```python
from build123d import *

# Parameters (mm, degrees)
F0_W     = 103.351444006
F0_H     = 32.4089471251
F0_R     = 8.8186134511
F2_DEPTH = 23.876
F3_T     = 2.54
F4_R     = 5.08
F5_DEPTH = 75.946
F6_DEPTH = 25.4


# Not quite as in the source:
# - a shell that OpenCascade refuses in one call is made with other operations: the cavity is built on its own and cut out
# - the program builds the solid bodies; features that only make, move or delete a surface that nothing else refers to are left out


with BuildPart() as f2:
    # F0 (on Front) → F2 (new body, symmetric)
    with BuildSketch(Plane.XZ):
        with Locations((-17.6653191447, -6.3865175471)):
            Rectangle(F0_W, F0_H)
        with Locations((-21.0040956736, 0)):
            Circle(F0_R, mode=Mode.SUBTRACT)
    extrude(amount=F2_DEPTH, both=True)

    # F3: shell of thickness 2.54, made by hand


with BuildPart() as f3_core1:
    # F3_t2: copy of F2
    add(f2.part)

    # the walls: a layer under each face that stays
    f3_faces = [f3_core1.faces().sort_by_distance(p)[0] for p in [
        (34.0104028583, 0, -6.3865175471),
        (-17.6653191447, 0, -22.5909911096),
        (-69.3410411477, 0, -6.3865175471),
        (-52.11580048, -23.876, -17.1894999221),
        (-29.8227091247, 0, 0),
        (-52.11580048, 23.876, -17.1894999221),
    ]]
    thicken(f3_faces, amount=-F3_T, mode=Mode.SUBTRACT)


with BuildPart() as f2_1:
    add(f2.part)

    # what is left inside the walls is the cavity
    f3_cavity = [f3_core1.part.solids().sort_by_distance(p)[0] for p in [
        (-17.665319, 7.112, -20.025591),
    ]]
    add(f3_cavity, mode=Mode.SUBTRACT)

    # F4
    f4_edges = [f2_1.edges().sort_by_distance(p)[0] for p in [
        (34.010403, 0, -22.590991),
    ]]
    fillet(f4_edges, radius=F4_R)

    # F5 (add): a face of the model
    f5_faces = [f2_1.faces().sort_by_distance(p)[0] for p in [
        (-18.9893309888, 0, 9.8179560155),
    ]]
    extrude(f5_faces, amount=F5_DEPTH)

    # F6 (add): a face of the model
    f6_faces = [f2_1.faces().sort_by_distance(p)[0] for p in [
        (-17.6163810634, -23.876, 32.3181446874),
    ]]
    extrude(f6_faces, amount=F6_DEPTH)

    # F7: F2 across plane


with BuildPart() as f2_2:
    add(f2_1.part)
    add(f2_1.part.mirror(Plane.YZ))


solid = f2_2.part
```
The listing builds one solid part. Answer for the finished solid, in the listing's coordinates (mm). A direction names the side the tool comes from. Coordinates: 2 decimals unless noted, no trailing zeros. Loops run counter-clockwise (first coordinate to the right, second up) from the corner with the lowest first, then second, coordinate; pieces in that order, holes last. Notation, with made-up numbers: M 84,59 L 110,59 A5 cw 110,67 Z; hole C 57.5,-33.75 d6. An arc over 180 degrees is marked long. Answer as CSV lines item,"result". Start each with the question number.
(1) The mould has two halves that part along Z. Classify faces 1 (the flat face through (-21, -21.336, 0)), 2 (the flat face through (1, -12, -22.591)), 3 (the flat face through (15.292, 0, 47)): pulls with the +Z half, pulls with the -Z half, needs draft (parallel to the pull), parting line crosses it, or undercut.
(2) The part is cut by section B-B (y = -4.5). State how many separate pieces and enclosed holes the cut face has, and give its area (3 significant figures).
(3) The part is cut by section A-A (z = 59). Give the vertices of the cut face in (x, y), and give its area (3 significant figures).
(4) Given pin 1 (21.5 mm diameter, centred on x = -2, y = 6, fed in from +Z); pin 2 (16.5 mm diameter, centred on x = 55.5, y = -2, fed in from +Z), each flat-ended and moving along its own axis, determine where each tip first touches the part or whether it passes through.
(5) Find the intervals of material crossed by L1, parallel to X at y = -8, z = 30; L2, parallel to Y at x = 0.5, z = 74.5; L3, parallel to Z at x = 13, y = -13.5, in increasing order. Write a range as [from, to].
(6) The part is cut by section D-D (z = 0). Give the vertices of the cut face in (x, y).
(7) For faces 4 (the flat face through (66.801, 0, 32)), 5 (the cylindrical face through (-29.814, 0.299, 0.388)), determine the directions among +Z, -Z, +X, -X, +Y, -Y from which every point of the face is accessible in a straight line to the end or side of a thin tool.
(8) The part is cut by section C-C (x = 40.5). Give the vertices of the cut face in (y, z), and give its area (3 significant figures).
Determined:
1,face 1,"undercut"
1,face 2,"pulls with the -Z half"
1,face 3,"needs draft"
2,separate pieces,"1"
2,enclosed holes,"2"
2,area,"3,450 mm2"
3,outline,"M -69.34,-49.28 L 69.34,-49.28 L 69.34,23.88 L -69.34,23.88 Z; hole M -66.8,-21.34 L -34.01,-21.34 L -34.01,21.34 L -66.8,21.34 Z; hole M -31.47,-21.34 L -26.72,-21.34 L -26.72,21.34 L -31.47,21.34 Z; hole M -15.29,-21.34 L 15.29,-21.34 L 15.29,21.34 L -15.29,21.34 Z; hole M 26.72,-21.34 L 31.47,-21.34 L 31.47,21.34 L 26.72,21.34 Z; hole M 34.01,-21.34 L 66.8,-21.34 L 66.8,21.34 L 34.01,21.34 Z"
3,area,"5,640 mm2"
4,pin 1,"z = 7.8"
4,pin 2,"z = -20.05"
5,L1,"[-69.34, -66.8], [-34.01, -31.47], [-26.72, -15.29], [15.29, 26.72], [31.47, 34.01], [66.8, 69.34]"
5,L2,"[-49.28, -21.34], [21.34, 23.88]"
5,L3,"[-22.59, -20.05], [-8.06, -3.7], [3.7, 8.06]"
6,outline,"M -69.34,-49.28 L 69.34,-49.28 L 69.34,23.88 L -69.34,23.88 Z; hole M -66.8,-21.34 L -34.01,-21.34 L -34.01,21.34 L -66.8,21.34 Z; hole M -29.82,-21.34 L -12.19,-21.34 L -12.19,21.34 L -29.82,21.34 Z; hole M -9.65,-21.34 L 9.65,-21.34 L 9.65,21.34 L -9.65,21.34 Z; hole M 12.19,-21.34 L 29.82,-21.34 L 29.82,21.34 L 12.19,21.34 Z; hole M 34.01,-21.34 L 66.8,-21.34 L 66.8,21.34 L 34.01,21.34 Z"
7,face 4,"+Z"
7,face 5,"none"
8,outline,"M -49.28,-22.59 L 23.88,-22.59 L 23.88,85.76 L 21.34,85.76 L 21.34,-20.05 L -21.34,-20.05 L -21.34,85.76 L -49.28,85.76 Z"
8,area,"3,410 mm2"
